Source: CAD feature listing. Evaluate the final solid. Frame: model axes, mm. Round coordinates to 2 decimals unless told otherwise and drop trailing zeros. Order: outer loops, then holes, each group sorted by start corner. A loop starts at its lowest first (then second) coordinate and runs counter-clockwise, first axis right, second up. Notation, with made-up numbers: (47.5, -13.75) -> (65.5, -13.75) arc R5 ccw to (65.5, -4.75) -> close; hole circle Ø11 at (76, -17). An arc over 180 degrees is marked (long way). Answer as CSV lines item,"result".
from build123d import *

# Parameters (mm, degrees)
F0_R     = 3.96875
F1_DEPTH = 4.7625
F2_R     = 6.35


# Not quite as in the source:
# - a feature names something its author has since deleted; it is built from what else it names


with BuildPart() as f1:
    # F0 (on Top) → F1 (new body)
    with BuildSketch(Plane.XY):
        with BuildLine():
            Line((31.8700148185, 7.8436681485), (15.5628504577, 88.8576204098))
            ThreePointArc((15.5628504577, 88.8576204098), (-0.5130479886, 101.5917074959), (-15.732715337, 87.8456822313))
            Line((-15.732715337, 87.8456822313), (-24.1670854724, 25.2735804658))
            Line((-24.1670854724, 25.2735804658), (-88.0768518519, 15.6998222241))
            ThreePointArc((-88.0768518519, 15.6998222241), (-101.6, 0), (-88.0768518519, -15.6998222241))
            Line((-88.0768518519, -15.6998222241), (-4.2333333333, -28.2596800033))
            ThreePointArc((-4.2333333333, -28.2596800033), (22.921010673, -19.3106758579), (31.8700148185, 7.8436681485))
        make_face()
        with Locations((-85.725, 0)):
            Circle(F0_R, mode=Mode.SUBTRACT)
        Circle(F0_R, mode=Mode.SUBTRACT)
        with Locations((0, 85.725)):
            Circle(F0_R, mode=Mode.SUBTRACT)
    extrude(amount=F1_DEPTH)

    # F2
    f2_edges = [f1.edges().sort_by_distance(p)[0] for p in [
        (-24.167085, 25.27358, 2.38125),
    ]]
    fillet(f2_edges, radius=F2_R)


solid = f1.part
1. Section query D-D on y = 38.5. Return loops of the section in (x, z), and give its area (3 significant figures).
Results below:
outline,"(-22.38, 0) -> (25.7, 0) -> (25.7, 4.76) -> (-22.38, 4.76) -> close"
area,"229 mm2"
2. Mould query, pull axis Y, two halves, no side actions, for faces 1 (the flat face through (-21, 23, 4.762)), 2 (the flat face through (23.83, 47.78, 2.35)), 3 (the cylindrical face through (-0.86, -3.874, 2.348)). Classes: released by +Y, released by -Y, zero draft, split by the parting line, or undercut.
Results below:
face 1,"zero draft"
face 2,"released by +Y"
face 3,"undercut"
3. Line query: L1, parallel to Y at x = 0, z = 3.85; L2, parallel to Y at x = -3.5, z = 3.2; L3, parallel to X at y = 30.5, z = 0.9. Output: solid intervals per line, ascending. Write a range as [from, to].
Results below:
L1,"[-28.61, -3.97], [3.97, 81.76], [89.69, 101.6]"
L2,"[-28.36, -1.87], [1.87, 83.85], [87.6, 101.21]"
L3,"[-23.46, 27.31]"
4. Pin query (flat end, axial travel): pin 1 (1 mm diameter, centred on x = -29.5, z = 2, fed in from -Y). Return the tip coordinate at first contact, or that it passes through.
Results below:
pin 1,"y = -24.55"
5. Section query C-C on x = 0. Return loops of the section in (y, z), and give its area (3 significant figures).
Results below:
outline,"(-28.61, 0) -> (-3.97, 0) -> (-3.97, 4.76) -> (-28.61, 4.76) -> close; (3.97, 0) -> (81.76, 0) -> (81.76, 4.76) -> (3.97, 4.76) -> close; (89.69, 0) -> (101.6, 0) -> (101.6, 4.76) -> (89.69, 4.76) -> close"
area,"545 mm2"
6. Section query B-B on y = 0. Return loops of the section in (x, z).
Results below:
outline,"(-101.6, 0) -> (-89.69, 0) -> (-89.69, 4.76) -> (-101.6, 4.76) -> close; (-81.76, 0) -> (-3.97, 0) -> (-3.97, 4.76) -> (-81.76, 4.76) -> close; (3.97, 0) -> (32.06, 0) -> (32.06, 4.76) -> (3.97, 4.76) -> close"
7. Section query A-A on z = 2.35. Give the number of separate pieces and of enclosed holes in the cut face, and give its area (3 significant figures).
Results below:
separate pieces,"1"
enclosed holes,"3"
area,"8,500 mm2"
